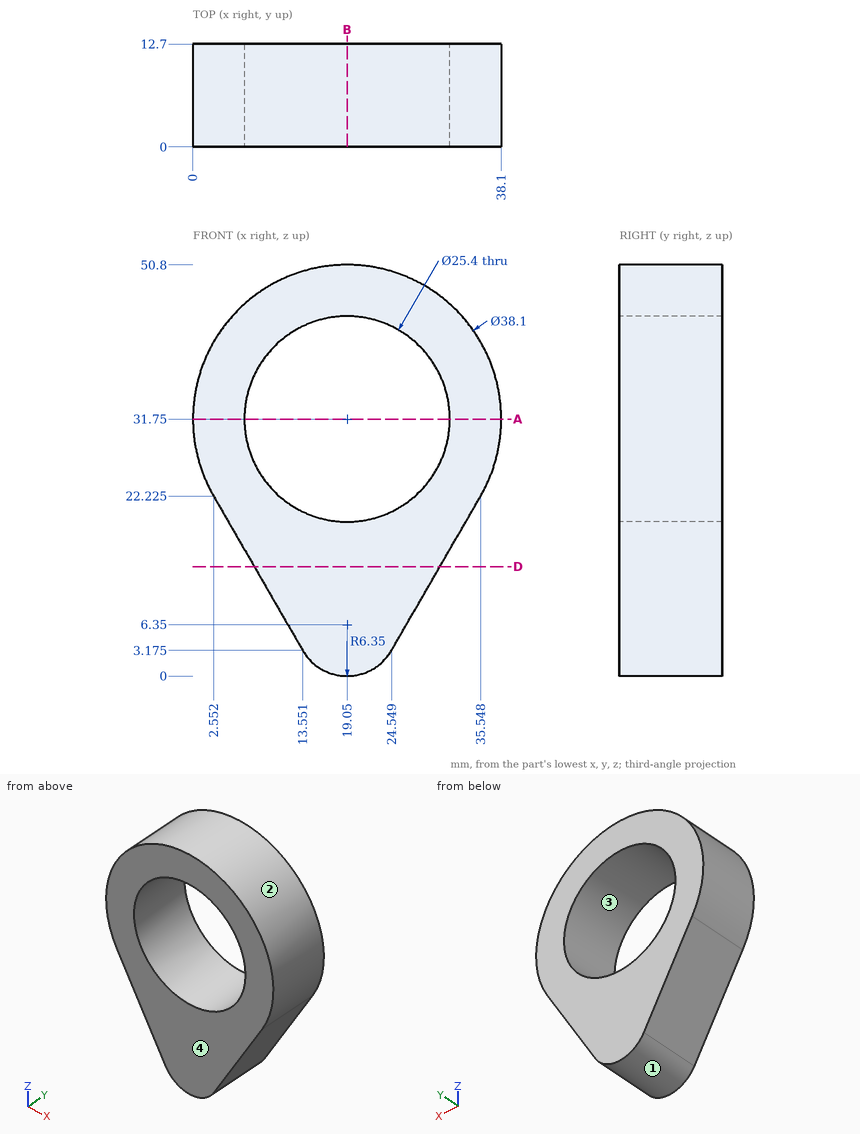
Design review of the part shown in the three views and the two pictorial views. Dimensions are in mm from the part's minimum x, y and z. Give positions to 0.01 mm unless a question says otherwise; leave off trailing zeros. Write each loop counter-clockwise with the first axis right and the second up, starting at its lowest first coordinate (ties: lowest second). Pieces come first, ordered by that corner, then holes.
Item 1: Take a section at A-A (z = 31.75). Give the boundary of the cut face in (x, y), and give its area (3 significant figures).
Item 2: Insertion check: P1, Ø2, axis at y = 3, z = 21, coming from the +X side; P2, Ø6, axis at x = 26, y = 5.5, coming from the +Z side; P3, Ø4, axis at y = 6.5, z = 15, coming from the -X side. Each pin has a flat end and moves straight along its axis. Give the tip position at first contact, or say it passes through.
Item 3: Take a section at D-D (z = 13.5). Give the boundary of the cut face in (x, y), and give its area (3 significant figures).
Item 4: Take a section at B-B (x = 19.05). Give the boundary of the cut face in (y, z), and give its area (3 significant figures).
Item 5: Wall thickness on probe 1 along Z at (x, y) = (23, 11.75) (1 decimal); probe 2 along X at (y, z) = (2, 24.5); probe 3 along X at (y, z) = (1.5, 36): over which ranges is each line inside the solid? List them lowest first.
Item 6: The part is to be moulded in two halves that separate along Z. For the marked faces 1, 2, 3 and 4, say which applies: +Z half, -Z half, draft (parallel to the pull), parting line (faces both ways), or undercut.
Established:
1. outline: (0, 0) - (6.35, 0) - (6.35, 12.7) - (0, 12.7) - close; (31.75, 0) - (38.1, 0) - (38.1, 12.7) - (31.75, 12.7) - close
1. area: 161 mm2
2. P1: stops at x = 35.42
2. P2: stops at z = 50.39
2. P3: stops at x = 5.57
3. outline: (7.59, 0) - (30.51, 0) - (30.51, 12.7) - (7.59, 12.7) - close
3. area: 291 mm2
4. outline: (0, 0) - (12.7, 0) - (12.7, 19.05) - (0, 19.05) - close; (0, 44.45) - (12.7, 44.45) - (12.7, 50.8) - (0, 50.8) - close
4. area: 323 mm2
5. probe 1: z = 1.4 to 19.7, 43.8 to 50.4
5. probe 2: x = 1.43 to 8.62, 29.48 to 36.67
5. probe 3: x = 0.48 to 7.08, 31.02 to 37.62
6. face 1: -Z half
6. face 2: parting line
6. face 3: undercut
6. face 4: draft
